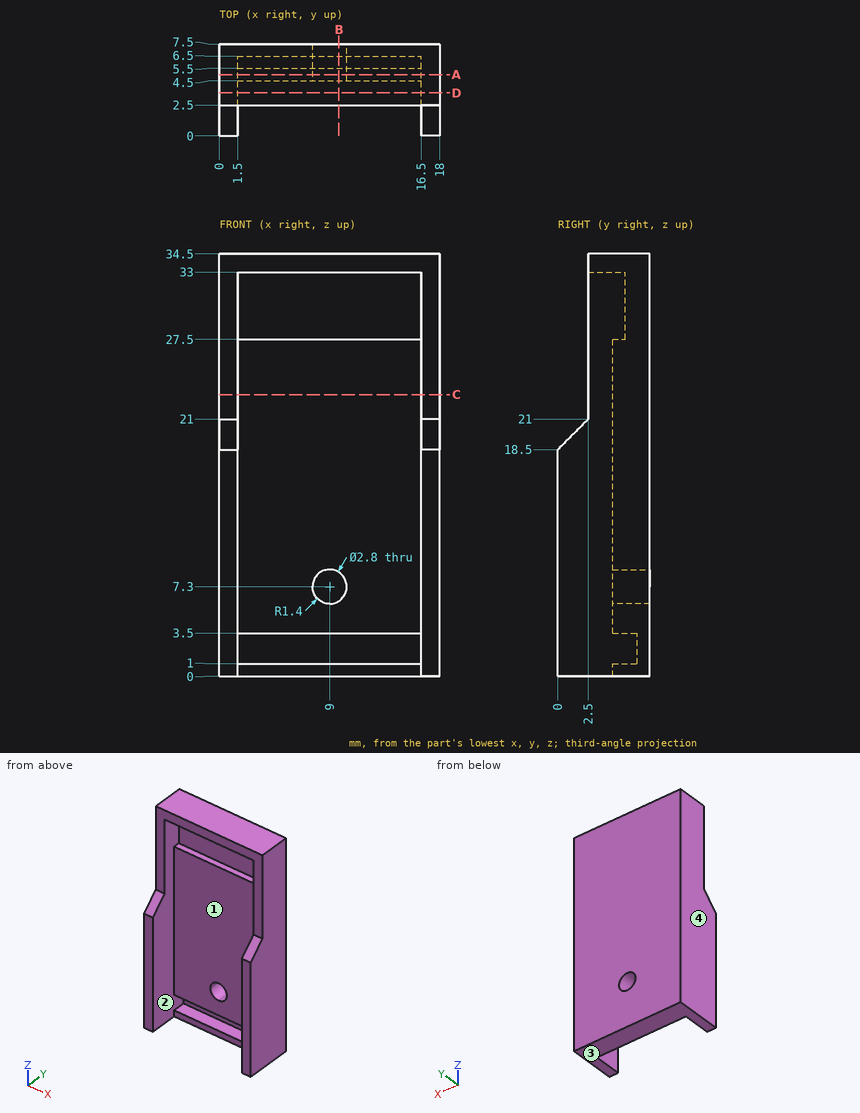
Can you work these out from the drawing? Everything is in mm from the part's minimum corner. Give positions to 0.01 mm unless a question says otherwise; leave off trailing zeros. Order: outer loops, then holes, each group sorted by start corner. A loop starts at its lowest first (then second) coordinate and runs counter-clockwise, first axis right, second up.
1. Will these pins go through, and if not, where does the flat tip stop? P1, Ø0.8, axis at x = 9.5, z = 0.5, coming from the -Y side; P2, Ø6, axis at x = 10, z = 31, coming from the -Y side; P3, Ø4, axis at x = 5.5, z = 30.5, coming from the -Y side.
2. Suppose I cut it at C-C (z = 23). List the corners of the cut face in (x, y) for me, plus the area to 3 significant figures.
3. Suppose I cut it at D-D (y = 3.5). List the corners of the cut face in (x, z) for me, plus the area to 3 significant figures.
4. I need wall thicknesses on L1, parallel to Z at x = 9, y = 5.8; L2, parallel to Z at x = 4.5, y = 4.75; L3, parallel to X at y = 6, z = 7.3. Which ranges of each line are inside material? Lowest first, please.
5. We'd pull the mould along X, two halves only. Please class the marked faces 1, 2, 3 and 4: pulls with the +X half, pulls with the -X half, needs draft (parallel to the pull), parting line crosses it, or undercut.
6. Suppose I cut it at A-A (y = 5). List the corners of the cut face in (x, z) for me.
7. Suppose I cut it at B-B (x = 9.75). List the corners of the cut face in (y, z) for me.
Solved:
1. P1: stops at y = 4.5
1. P2: stops at y = 2.5
1. P3: stops at y = 5.5
2. outline: (0, 2.5) - (1.5, 2.5) - (1.5, 4.5) - (16.5, 4.5) - (16.5, 2.5) - (18, 2.5) - (18, 7.5) - (0, 7.5) - close
2. area: 60.0 mm2
3. outline: (0, 0) - (1.5, 0) - (1.5, 33) - (16.5, 33) - (16.5, 0) - (18, 0) - (18, 34.5) - (0, 34.5) - close
3. area: 126 mm2
4. L1: z = 0 to 1, 3.5 to 5.9, 8.7 to 34.5
4. L2: z = 0 to 1, 3.5 to 27.5, 33 to 34.5
4. L3: x = 0 to 7.6, 10.4 to 18
5. face 1: undercut
5. face 2: undercut
5. face 3: needs draft
5. face 4: pulls with the -X half
6. outline: (0, 0) - (18, 0) - (18, 34.5) - (0, 34.5) - close; hole (1.5, 1) - (16.5, 1) - (16.5, 3.5) - (1.5, 3.5) - close; hole (1.5, 27.5) - (16.5, 27.5) - (16.5, 33) - (1.5, 33) - close; hole circle Ø2.8 at (9, 7.3)
7. outline: (2.5, 33) - (5.5, 33) - (5.5, 27.5) - (4.5, 27.5) - (4.5, 8.48) - (7.5, 8.48) - (7.5, 34.5) - (2.5, 34.5) - close; (4.5, 0) - (7.5, 0) - (7.5, 6.12) - (4.5, 6.12) - (4.5, 3.5) - (6.5, 3.5) - (6.5, 1) - (4.5, 1) - close
